Input: part model. Units: mm. Frame: model coordinates. Coordinates: 2 decimals unless noted, no trailing zeros. Order: outer loops, then holes, each group sorted by start corner. A loop starts at its lowest first (then second) coordinate and runs counter-clockwise, first axis right, second up. Notation, with made-up numbers: (-21.5, 27.25) -> (19.5, 27.25) arc R17 cw to (19.5, 47.25) -> close; hole circle Ø11 at (25, 51.5). An arc over 180 degrees is marked (long way). One line per item, written item: value. Start each with the question number.
from build123d import *

# Parameters (mm, degrees)
F1_DEPTH = 7.5
F6_D     = 4.24


with BuildPart() as f4:
    # F0 (on Right) → F4 (revolve)
    with BuildSketch(Plane.YZ):
        with BuildLine():
            Line((-7.5, 0), (0, 0))
            Line((0, 0), (6.288552845, 0))
            add(Edge.make_bspline(
                [(6.288552845, 0), (6.2874522314, 4.9991249071), (0, 5)],
                knots=[0.0004759058, 0.0004759058, 0.0004759058, 1.5710971834, 1.5710971834, 1.5710971834], degree=2, weights=[1, 0.7071686677, 1]))
            Line((0, 5), (-0.0011008063, 5))
            Line((-0.0011008063, 5), (-7.5, 5))
            Line((-7.5, 5), (-7.5, 0))
        make_face()
    revolve(axis=Axis((0, -3.8328841329, 0), (0, 1, 0)))

    # F5 (on face) → F1 (join)
    with BuildSketch(Plane.XZ.offset(7.5)):
        Polygon((5.8867447078, 3.3254646696), (0, 7.0603471249), (-5.8867447078, 3.3254646696), (-5.8867447078, -3.6461284202), (0, -7.3810108755), (5.8867447078, -3.6461284202), align=None)
    extrude(amount=-F1_DEPTH)

    # F6 (through all)
    with Locations(Plane.XZ.offset(7.5)):
        with Locations((0, 0)):
            Hole(F6_D / 2)


solid = f4.part
1) Mould query, pull axis Z, two halves, no side actions, for faces 1 (the flat face through (-2, 0, -5)), 2 (the cylindrical face through (-2.02, -0.81, 0.64)), 3 (the flat face through (2.9, -3.8, -5.54)). Classes: +Z half, -Z half, draft (parallel to the pull), parting line (faces both ways), or undercut.
2) Section query B-B, the plane z = 6. Return the cut outline in (x, y).
3) Pin query (flat end, axial travel): pin 1 Ø4 at (x, z) = (0, 0) entering from -Y; pin 2 Ø1.5 at (x, z) = (-0.5, 3) entering from +Y; pin 3 Ø4 at (x, z) = (3, -5.5) entering from +Y. Return the tip coordinate at first contact, or that it passes through.
4) Section query A-A, the plane y = -5.75. Return the cut outline in (x, z).
5) Ray query, line 1 along X through (y, z) = (-0.25, 0); line 2 along Y through (x, z) = (-0.5, -5.5); line 3 along Z through (x, y) = (0.75, -4). Return the intervals inside material, ascending. Write a range as from..to.
Entries:
1. face 1: draft
1. face 2: undercut
1. face 3: -Z half
2. outline: (-1.67, -7.5) -> (1.67, -7.5) -> (1.67, 0) -> (-1.67, 0) -> close
3. pin 1: passes through
3. pin 2: stops at y = 5.59
3. pin 3: stops at y = 3.28
4. outline: (-5.89, -3.65) -> (0, -7.38) -> (5.89, -3.65) -> (5.89, 3.33) -> (0, 7.06) -> (-5.89, 3.33) -> close; hole circle Ø4.24 at (0, 0)
5. line 1: x = -5.89..-2.12, 2.12..5.89
5. line 2: y = -7.5..0
5. line 3: z = -6.91..-1.98, 1.98..6.58
